from build123d import *

# Parameters (mm, degrees)
BOSS_EXTRUDE1_DEPTH = 6.35
BOSS_EXTRUDE2_DEPTH = 11.43
CUT_EXTRUDE1_DEPTH  = 12.7
FILLET1_R           = 2.54


with BuildPart() as part:
    # Sketch1 → Boss-Extrude1 (new body)
    with BuildSketch(Plane(origin=(0, 0, 0), x_dir=(1, 0, 0), z_dir=(0, 1, 0))):
        Polygon((0, 0), (0, 76.2), (88.9, 76.2), (88.9, 127), (266.7, 127), (266.7, 0), align=None)
    extrude(amount=BOSS_EXTRUDE1_DEPTH)

    # Sketch2 → Boss-Extrude2 (add)
    with BuildSketch(Plane(origin=(0, 6.35, 0), x_dir=(1, 0, 0), z_dir=(0, 1, 0))):
        Polygon((19.05, 63.5), (101.6, 63.5), (101.6, 107.95), (88.9, 107.95), (88.9, 76.2), (19.05, 76.2), align=None)
    extrude(amount=-BOSS_EXTRUDE2_DEPTH)

    # Sketch3 → Cut-Extrude1 (cut)
    with BuildSketch(Plane(origin=(0, 6.35, 0), x_dir=(1, 0, 0), z_dir=(0, 1, 0))):
        Polygon((235.204, 31.496), (235.204, 52.324), (227.076, 49.784), (227.076, 34.036), align=None)
    extrude(amount=-CUT_EXTRUDE1_DEPTH, mode=Mode.SUBTRACT)

    # Fillet1
    fillet1_edges = [part.edges().sort_by_distance(p)[0] for p in [
        (235.204, 3.175, -31.496),
        (227.076, 3.175, -34.036),
        (227.076, 3.175, -49.784),
        (235.204, 3.175, -52.324),
    ]]
    fillet(fillet1_edges, radius=FILLET1_R)


solid = part.part
CAD build for the part. Positions are in the model's coordinates, mm. A direction names the side the tool comes from. Round coordinates to 2 decimals unless told otherwise and drop trailing zeros. Write each loop counter-clockwise with the first axis right and the second up, starting at its lowest first coordinate (ties: lowest second). Pieces come first, ordered by that corner, then holes.
(1) Slice it at C-C, the plane x = 86.5. Write the cut outline in (y, z), and give its area (3 significant figures).
(2) Slice it at A-A, the plane y = 2.5. Write the cut outline in (x, z), and give its area (3 significant figures).
(3) Drop flat-ended pins along their axis: P1, Ø5, axis at x = 29, z = -58.5, coming from the -Y side; P2, Ø1.5, axis at x = 80, y = -2, coming from the +Z side; P3, Ø3.5, axis at y = 3.5, z = -95.5, coming from the -X side. Give the stop position or say it passes through.
(4) Slice it at D-D, the plane z = -104.5. Write the cut outline in (x, y), and give its area (3 significant figures).
(5) 3-axis set-ups, long thin cutter, end or side, ignore diameter. For faces 1 (the face through (95, -3, -107.95)), 2 (the face through (19.05, -3, -70)), 3 (the face through (235.204, 3, -42)): which of +Z, -Z, +X, -X, +Y, -Y reach the whole face in a straight line?
(6) Mould opens along Z. For faces 4 (the face through (227.076, 3, -42)), 5 (the face through (44, 1, -76.2)), 6 (the face through (88.9, 1, -96)) say: pulls with the +Z half, pulls with the -Z half, needs draft (parallel to the pull), parting line crosses it, or undercut.
(7) Probe line 1 along X through (y, z) = (5, -43); line 2 along X through (y, z) = (-3, -74.5); line 3 along Y through (x, z) = (248, -87). List the from-to ranges inside material, lowest first.
(8) Slice it at B-B, the plane z = -70. Write the cut outline in (x, y), and give its area (3 significant figures).
From the geometry:
1. outline: (-5.08, -76.2) - (6.35, -76.2) - (6.35, 0) - (0, 0) - (0, -63.5) - (-5.08, -63.5) - close
1. area: 548 mm2
2. outline: (0, -76.2) - (88.9, -76.2) - (88.9, -127) - (266.7, -127) - (266.7, 0) - (0, 0) - close; hole (227.08, -47.92) arc R2.54 ccw to (228.86, -50.34) - (231.91, -51.29) arc R2.54 ccw to (235.2, -48.87) - (235.2, -34.95) arc R2.54 ccw to (231.91, -32.53) - (228.86, -33.48) arc R2.54 ccw to (227.08, -35.9) - close
2. area: 29,200 mm2
3. P1: stops at y = 0
3. P2: stops at z = -63.5
3. P3: stops at x = 88.9
4. outline: (88.9, -5.08) - (101.6, -5.08) - (101.6, 0) - (266.7, 0) - (266.7, 6.35) - (88.9, 6.35) - close
4. area: 1,190 mm2
5. face 1: -Z, +X, -X, -Y
5. face 2: +Z, -Z, -X, -Y
5. face 3: +Y, -Y
6. face 4: undercut
6. face 5: pulls with the -Z half
6. face 6: needs draft
7. line 1: x = 0 to 227.08, 235.2 to 266.7
7. line 2: x = 19.05 to 101.6
7. line 3: y = 0 to 6.35
8. outline: (0, 0) - (19.05, 0) - (19.05, -5.08) - (101.6, -5.08) - (101.6, 0) - (266.7, 0) - (266.7, 6.35) - (0, 6.35) - close
8. area: 2,110 mm2
